```python
from build123d import *

# Parameters (mm, degrees)
SKETCH1_R           = 3.7
BOSS_EXTRUDE1_DEPTH = 8
FILLET1_R           = 10
SKETCH2_W           = 10
SKETCH2_H           = 127
BOSS_EXTRUDE2_DEPTH = 30
BOSS_EXTRUDE3_DEPTH = 7
FILLET2_R           = 3
SKETCH4_W           = 18
SKETCH4_H           = 8
BOSS_EXTRUDE4_DEPTH = 27
SKETCH5_W           = 25
SKETCH5_H           = 8
BOSS_EXTRUDE5_DEPTH = 33
SKETCH6_W           = 25
SKETCH6_H           = 23.005701243
BOSS_EXTRUDE6_DEPTH = 8
SKETCH7_W           = 25
SKETCH7_H           = 7.5
BOSS_EXTRUDE7_DEPTH = 15
CUT_EXTRUDE1_REACH  = 159.817
SKETCH8_R           = 1.6
FILLET3_R           = 8
FILLET4_R           = 5
CUT_EXTRUDE2_REACH  = 163.149
SKETCH9_W           = 8
SKETCH9_H           = 5.5
FILLET7_R           = 3
BOSS_EXTRUDE8_DEPTH = 10
CUT_EXTRUDE3_START  = -17.777833
CUT_EXTRUDE3_DEPTH  = 17.777833


with BuildPart() as part:
    # Sketch1 → Boss-Extrude1 (new body)
    with BuildSketch(Plane(origin=(0, 0, 0), x_dir=(1, 0, 0), z_dir=(0, 1, 0))):
        with BuildLine():
            Line((0, 0), (0, -140))
            Line((0, -140), (6, -150))
            Line((6, -150), (13.995477091, -150))
            ThreePointArc((13.995477091, -150), (23.898170207, -145.898170207), (28, -135.995477091))
            Line((28, -135.995477091), (28, 0))
            Line((28, 0), (0, 0))
        make_face()
        with Locations(Location((10, -135, 0), (0, 0, 270))):
            Circle(SKETCH1_R, mode=Mode.SUBTRACT)
    extrude(amount=BOSS_EXTRUDE1_DEPTH)

    # Fillet1
    fillet1_edges = [part.edges().sort_by_distance(p)[0] for p in [
        (6, 4, 150),
        (0, 4, 140),
    ]]
    fillet(fillet1_edges, radius=FILLET1_R)

    # Sketch2 → Boss-Extrude2 (add)
    with BuildSketch(Plane(origin=(0, 8, 0), x_dir=(1, 0, 0), z_dir=(0, 1, 0))):
        with Locations((23, -63.5)):
            Rectangle(SKETCH2_W, SKETCH2_H)
    extrude(amount=BOSS_EXTRUDE2_DEPTH)

    # Sketch3 → Boss-Extrude3 (add)
    with BuildSketch(Plane(origin=(0, 38, 0), x_dir=(1, 0, 0), z_dir=(0, 1, 0))):
        with BuildLine():
            Line((18, 0), (38, 0))
            Line((38, 0), (38, -106.265006005))
            ThreePointArc((38, -106.265006005), (34.694156342, -131.484540297), (25, -155))
            Line((25, -155), (18, -127))
            Line((18, -127), (18, 0))
        make_face()
    extrude(amount=BOSS_EXTRUDE3_DEPTH)

    # Fillet2
    fillet2_edges = [part.edges().sort_by_distance(p)[0] for p in [
        (0, 4, 0),
        (18, 26.5, 0),
        (25, 41.5, 155),
    ]]
    fillet(fillet2_edges, radius=FILLET2_R)

    # Sketch4 → Boss-Extrude4 (add)
    with BuildSketch(Plane(origin=(0, 8, 0), x_dir=(1, 0, 0), z_dir=(0, 1, 0))):
        with Locations((9, -21.010298757)):
            Rectangle(SKETCH4_W, SKETCH4_H)
        with Locations((9, -81.507298757)):
            Rectangle(SKETCH4_W, SKETCH4_H)
    extrude(amount=BOSS_EXTRUDE4_DEPTH)

    # Sketch5 → Boss-Extrude5 (add)
    with BuildSketch(Plane(origin=(0, 35, 0), x_dir=(1, 0, 0), z_dir=(0, 1, 0))):
        with Locations((12.5, -21.010298757)):
            Rectangle(SKETCH5_W, SKETCH5_H)
        with Locations((12.5, -81.507298757)):
            Rectangle(SKETCH5_W, SKETCH5_H)
    extrude(amount=BOSS_EXTRUDE5_DEPTH)

    # Sketch6 → Boss-Extrude6 (add)
    with BuildSketch(Plane(origin=(0, 68, 0), x_dir=(1, 0, 0), z_dir=(0, 1, 0))):
        with Locations((12.5, -89.010149379)):
            Rectangle(SKETCH6_W, SKETCH6_H)
    extrude(amount=BOSS_EXTRUDE6_DEPTH)

    # Sketch7 → Boss-Extrude7 (add)
    with BuildSketch(Plane.XY.offset(85.507298757)):
        with Locations((12.5, 48.75)):
            Rectangle(SKETCH7_W, SKETCH7_H)
    extrude(amount=BOSS_EXTRUDE7_DEPTH)

    # Sketch8 → Cut-Extrude1 (cut, up to next)
    with BuildSketch(Plane(origin=(0, 0, 17.010298757), x_dir=(-1, 0, 0), z_dir=(0, 0, -1)), mode=Mode.PRIVATE) as cut_extrude1_sk1:
        with Locations((-20, 60.5)):
            Circle(SKETCH8_R)
    cut_extrude1_tool1 = extrude(cut_extrude1_sk1.sketch, amount=-CUT_EXTRUDE1_REACH, mode=Mode.PRIVATE) & part.part
    # Sketch8 → Cut-Extrude1 (cut, up to next)
    with BuildSketch(Plane(origin=(0, 0, 17.010298757), x_dir=(-1, 0, 0), z_dir=(0, 0, -1)), mode=Mode.PRIVATE) as cut_extrude1_sk2:
        with Locations((-5, 60.5)):
            Circle(SKETCH8_R)
    cut_extrude1_tool2 = extrude(cut_extrude1_sk2.sketch, amount=-CUT_EXTRUDE1_REACH, mode=Mode.PRIVATE) & part.part
    add(cut_extrude1_tool1.solids().sort_by_distance((20, 60.5, 17.010299))[0], mode=Mode.SUBTRACT)
    add(cut_extrude1_tool2.solids().sort_by_distance((5, 60.5, 17.010299))[0], mode=Mode.SUBTRACT)

    # Fillet3
    fillet3_edges = [part.edges().sort_by_distance(p)[0] for p in [
        (18.878679656, 8, 0.878679656),
        (18, 8, 10.005149379),
    ]]
    fillet(fillet3_edges, radius=FILLET3_R)
    fillet3_2_edges = [part.edges().sort_by_distance(p)[0] for p in [
        (5, 8, 17.010298757),
    ]]
    fillet(fillet3_2_edges, radius=FILLET3_R)
    fillet3_3_edges = [part.edges().sort_by_distance(p)[0] for p in [
        (21.5, 45, 17.010298757),
    ]]
    fillet(fillet3_3_edges, radius=FILLET3_R)
    fillet3_4_edges = [part.edges().sort_by_distance(p)[0] for p in [
        (18, 26.5, 25.010298757),
    ]]
    fillet(fillet3_4_edges, radius=FILLET3_R)
    fillet3_5_edges = [part.edges().sort_by_distance(p)[0] for p in [
        (5, 8, 25.010298757),
    ]]
    fillet(fillet3_5_edges, radius=FILLET3_R)
    fillet3_6_edges = [part.edges().sort_by_distance(p)[0] for p in [
        (21.5, 45, 25.010298757),
    ]]
    fillet(fillet3_6_edges, radius=FILLET3_R)
    fillet3_7_edges = [part.edges().sort_by_distance(p)[0] for p in [
        (5, 8, 77.507298757),
    ]]
    fillet(fillet3_7_edges, radius=FILLET3_R)
    fillet3_8_edges = [part.edges().sort_by_distance(p)[0] for p in [
        (21.5, 45, 77.507298757),
    ]]
    fillet(fillet3_8_edges, radius=FILLET3_R)
    fillet3_9_edges = [part.edges().sort_by_distance(p)[0] for p in [
        (9, 8, 85.507298757),
    ]]
    fillet(fillet3_9_edges, radius=FILLET3_R)
    fillet3_10_edges = [part.edges().sort_by_distance(p)[0] for p in [
        (18, 30.5, 85.507298757),
    ]]
    fillet(fillet3_10_edges, radius=FILLET3_R)

    # Fillet4
    fillet4_edges = [part.edges().sort_by_distance(p)[0] for p in [
        (38, 41.5, 0),
        (25, 68, 21.010298757),
        (25, 76, 89.010149379),
        (0, 76, 89.010149379),
        (0, 68, 21.010298757),
        (12.5, 76, 100.513),
        (25, 72, 100.513),
        (0, 72, 100.513),
        (25, 48.75, 100.507298757),
        (0, 48.75, 100.507298757),
    ]]
    fillet(fillet4_edges, radius=FILLET4_R)

    # Sketch9 → Cut-Extrude2 (cut, up to next)
    with BuildSketch(Plane(origin=(0, 45, 0), x_dir=(1, 0, 0), z_dir=(0, 1, 0)), mode=Mode.PRIVATE) as cut_extrude2_sk1:
        with Locations((34, -12.754149379)):
            Rectangle(SKETCH9_W, SKETCH9_H)
    cut_extrude2_tool1 = extrude(cut_extrude2_sk1.sketch, amount=-CUT_EXTRUDE2_REACH, mode=Mode.PRIVATE) & part.part
    add(cut_extrude2_tool1.solids().sort_by_distance((34, 45, 12.754149))[0], mode=Mode.SUBTRACT)

    # Fillet7
    fillet7_edges = [part.edges().sort_by_distance(p)[0] for p in [
        (38, 41.5, 10.004149379),
        (38, 41.5, 15.504149379),
    ]]
    fillet(fillet7_edges, radius=FILLET7_R)

    # Sketch10 → Boss-Extrude8 (add)
    with BuildSketch(Plane.XZ.offset(-38)):
        with BuildLine():
            Line((18, 127), (28, 127))
            Line((28, 127), (35.777833095, 127))
            ThreePointArc((35.777833095, 127), (32.833324538, 137.640533241), (28.708897726, 147.881635807))
            ThreePointArc((28.708897726, 147.881635807), (25.702724236, 149.591554326), (23.08332777, 147.333311082))
            Line((23.08332777, 147.333311082), (18, 127))
        make_face()
    extrude(amount=BOSS_EXTRUDE8_DEPTH)

    # Sketch11 → Cut-Extrude3 (cut)
    with BuildSketch(Plane.ZY.offset(-18).offset(CUT_EXTRUDE3_START)):
        Polygon((127, 28), (127, 38), (149.605704206, 30.5), (149.605704206, 28), align=None)
        Polygon((149.605704206, 45), (149.605704206, 37.5), (127, 45), align=None)
    extrude(amount=CUT_EXTRUDE3_DEPTH, mode=Mode.SUBTRACT)


solid = part.part
```
Part model, mm, in its own coordinate system. A direction names the side the tool comes from. Coordinates: 2 decimals unless noted, no trailing zeros. Write each loop counter-clockwise with the first axis right and the second up, starting at its lowest first coordinate (ties: lowest second). Pieces come first, ordered by that corner, then holes.
Item 1: Mould opens along Z. For faces 1 (the face through (23.5, 48.8, 99.08)), 2 (the face through (10.163, 3.944, 131.304)), 3 (the face through (24, 17, 0)) say: released by +Z, released by -Z, zero draft, split by the parting line, or undercut.
Item 2: Slice it at C-C (z = 117.5). Write the cut outline in (x, y), and give its area (3 significant figures).
Item 3: Pin check, flat tips, straight feed: pin 1 (2 mm diameter, centred on x = 24.5, y = 25.5, fed in from +Z); pin 2 (2.5 mm diameter, centred on x = 32.5, y = 41, fed in from +Z); pin 3 (8.5 mm diameter, centred on y = 24, z = 46, fed in from -X). Stop position of each tip, or through.
Item 4: Slice it at B-B (y = 19). Write the cut outline in (x, z).
Item 5: Probe line 1 (Y direction, x = 5, z = 19); line 2 (X direction, y = 60, z = 22); line 3 (Z direction, x = 3.5, y = 34.5). List the from-to ranges inside material, lowest first.
Item 6: Which spindle directions (+Z, -Z, +X, -X, +Y, -Y) get a long thin tool onto all of the face, cutting with end or side? Do faces 4 (the face through (37.098, 41.451, 9.149)), 5 (the face through (5.07, 10.281, 87.913)), 6 (the face through (28, 19, 69)), 7 (the face through (2, 67, 21)), 8 (the face through (15.59, 30.65, 27.29)). Say none if no direction does.
Item 7: Slice it at A-A (y = 60.5). Write the cut outline in (x, z).
Results found:
1. face 1: released by +Z
1. face 2: undercut
1. face 3: released by -Z
2. outline: (0, 0) - (28, 0) - (28, 38) - (37.35, 38) - (37.35, 45) - (18, 45) - (18, 16) arc R8 cw to (10, 8) - (0, 8) - close
2. area: 673 mm2
3. pin 1: stops at z = 127
3. pin 2: stops at z = 141.33
3. pin 3: stops at x = 18
4. outline: (0, 17.01) - (10, 17.01) arc R8 cw to (18, 9.01) - (18, 3) arc R3 ccw to (21, 0) - (28, 0) - (28, 127) - (18, 127) - (18, 93.51) arc R8 cw to (10, 85.51) - (0, 85.51) - (0, 77.51) - (10, 77.51) arc R8 cw to (18, 69.51) - (18, 33.01) arc R8 cw to (10, 25.01) - (0, 25.01) - close
5. line 1: y = 0 to 58.9, 62.1 to 68
5. line 2: x = 0 to 3.48, 6.52 to 18.48, 21.52 to 25
5. line 3: z = 17.01 to 25.01, 77.51 to 85.51
6. face 4: +X, +Y, -Y
6. face 5: +Z, -X
6. face 6: -Z, +X, -Y
6. face 7: -Z, -X, +Y
6. face 8: -X, +Y
7. outline: (0, 17.01) - (3.4, 17.01) - (3.4, 25.01) - (0, 25.01) - close; (0, 77.51) - (25, 77.51) - (25, 85.51) - (0, 85.51) - close; (6.6, 17.01) - (18.4, 17.01) - (18.4, 25.01) - (6.6, 25.01) - close; (21.6, 17.01) - (25, 17.01) - (25, 25.01) - (21.6, 25.01) - close
